Part model, mm, in its own coordinate system. Coordinates: 2 decimals unless noted, no trailing zeros. Loops run counter-clockwise (first coordinate to the right, second up) from the corner with the lowest first, then second, coordinate; pieces in that order, holes last.
```python
from build123d import *

# Parameters (mm, degrees)
PROFILE_SKETCH_W          = 2.5
PROFILE_SKETCH_H          = 18.3
PROFILE_EXTRUDE_DEPTH     = 88
COVER_LATCH_CUT_OUT_DEPTH = 2.25
SIDE_SKETCH_W             = 0.25
SIDE_SKETCH_H             = 18.3
SIDE_EXTRUDE_DEPTH        = 88


with BuildPart() as part:
    # Profile Sketch → Profile Extrude (new body)
    with BuildSketch(Plane(origin=(0.045617437, 0, -0.024209872), x_dir=(-1, 0, 0), z_dir=(0, 1, 0))):
        with Locations((1.295617437, -9.125790128)):
            Rectangle(PROFILE_SKETCH_W, PROFILE_SKETCH_H)
    extrude(amount=PROFILE_EXTRUDE_DEPTH)

    # Cover Latch Cut Out Sketch → Cover Latch Cut Out (cut)
    with BuildSketch(Plane.ZY.offset(2.5)):
        Polygon((-18.3, 27), (-18.3, 13), (-8.858262488, 13), (-8.858262488, 5), (0, 5), (0, 15), (-2.2, 15), (-2.858262488, 20), (-2.2, 25), (0, 25), (0, 35), (-8.858262488, 35), (-8.858262488, 27), align=None)
    cover_latch_cut_out = extrude(amount=-COVER_LATCH_CUT_OUT_DEPTH, mode=Mode.SUBTRACT)

    # Cover Latch Cut Out Mirror: Cover Latch Cut Out across plane
    add(cover_latch_cut_out.mirror(Plane(origin=(0, 44, 0), x_dir=(0, 0, 1), z_dir=(0, -1, 0))), mode=Mode.SUBTRACT)

    # Side Sketch → Side Extrude (add, through all)
    with BuildSketch(Plane(origin=(0, 0, 0), x_dir=(1, 0, 0), z_dir=(0, 1, 0))):
        with Locations((-2.625, 9.15)):
            Rectangle(SIDE_SKETCH_W, SIDE_SKETCH_H)
    extrude(amount=SIDE_EXTRUDE_DEPTH)


solid = part.part
```
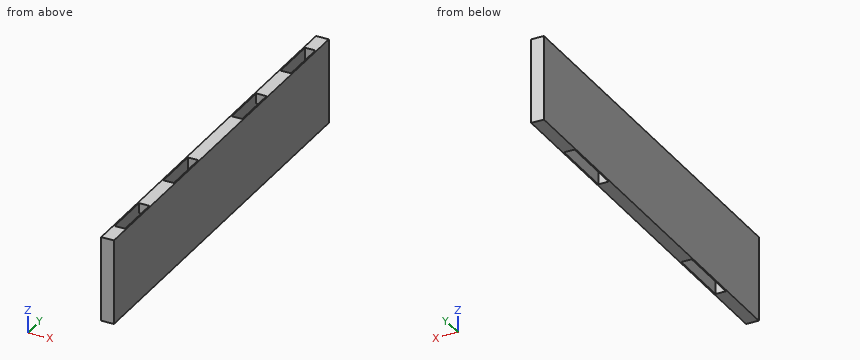
Q1. Probe line 1 (Y direction, x = -1.5, z = -7.5); line 2 (Y direction, x = -1.3, z = -11.25); line 3 (Y direction, x = -2, z = -1.5). List the from-to ranges inside material, lowest first.
Q2. Saw through at C-C (z = -1). List the corners of the cut face in (x, y).
Q3. Drop a flat-ended pin along its axis: P1, Ø0.7, axis at x = -2, z = -0.5, coming from the -Y side. Give the stop position or say it passes through.
Q4. Saw through at D-D (y = 76). List the corners of the cut face in (x, z).
Q5. Saw through at A-A (x = -1.15). Count the separate pieces of the cut face and the enclosed holes in it, plus the area to 3 significant figures.
Q6. Saw through at B-B (z = -15.5). List the corners of the cut face in (x, y), plus the area to 3 significant figures.
Checked values:
1. line 1: y = 0 to 5, 35 to 53, 83 to 88
1. line 2: y = 0 to 13, 27 to 61, 75 to 88
1. line 3: y = 0 to 5, 15 to 25, 35 to 53, 63 to 73, 83 to 88
2. outline: (-2.75, 0) - (0, 0) - (0, 88) - (-2.75, 88) - close; hole (-2.5, 5) - (-0.25, 5) - (-0.25, 15) - (-2.5, 15) - close; hole (-2.5, 25) - (-0.25, 25) - (-0.25, 35) - (-2.5, 35) - close; hole (-2.5, 53) - (-0.25, 53) - (-0.25, 63) - (-2.5, 63) - close; hole (-2.5, 73) - (-0.25, 73) - (-0.25, 83) - (-2.5, 83) - close
3. P1: stops at y = 0
4. outline: (-2.75, -18.3) - (0, -18.3) - (0, 0) - (-0.25, 0) - (-0.25, -8.86) - (-2.5, -8.86) - (-2.5, 0) - (-2.75, 0) - close
5. separate pieces: 5
5. enclosed holes: 0
5. area: 865 mm2
6. outline: (-2.75, 0) - (0, 0) - (0, 88) - (-2.75, 88) - close; hole (-2.5, 13) - (-0.25, 13) - (-0.25, 27) - (-2.5, 27) - close; hole (-2.5, 61) - (-0.25, 61) - (-0.25, 75) - (-2.5, 75) - close
6. area: 179 mm2
